Verification items for the finished model (mm, model axes). Face numbers are marked on the shaded views. Coordinates: 2 decimals unless noted, no trailing zeros. Write each loop counter-clockwise with the first axis right and the second up, starting at its lowest first coordinate (ties: lowest second). Pieces come first, ordered by that corner, then holes.
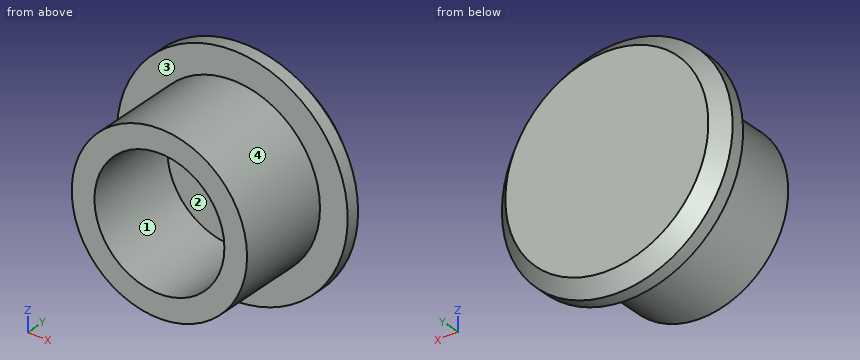
```python
from build123d import *

# Parameters (mm, degrees)
SKETCH1_R           = 6.33
BOSS_EXTRUDE1_DEPTH = 7
SKETCH2_R           = 4.691712698
CUT_EXTRUDE1_DEPTH  = 7
SKETCH3_R           = 8.33
BOSS_EXTRUDE2_DEPTH = 2
CHAMFER1_SIZE       = 1


with BuildPart() as part:
    # Sketch1 → Boss-Extrude1 (new body)
    with BuildSketch(Plane(origin=(0, 0, 0), x_dir=(1, 0, 0), z_dir=(0, 1, 0))):
        Circle(SKETCH1_R)
    extrude(amount=BOSS_EXTRUDE1_DEPTH)

    # Sketch2 → Cut-Extrude1 (cut)
    with BuildSketch(Plane(origin=(0, 7, 0), x_dir=(1, 0, 0), z_dir=(0, 1, 0))):
        Circle(SKETCH2_R)
    extrude(amount=-CUT_EXTRUDE1_DEPTH, mode=Mode.SUBTRACT)

    # Sketch3 → Boss-Extrude2 (add)
    with BuildSketch(Plane(origin=(0, 7, 0), x_dir=(1, 0, 0), z_dir=(0, 1, 0))):
        Circle(SKETCH3_R)
    extrude(amount=BOSS_EXTRUDE2_DEPTH)

    # Chamfer1
    chamfer1_edges = [part.edges().sort_by_distance(p)[0] for p in [
        (-8.33, 9, 0),
    ]]
    chamfer(chamfer1_edges, length=CHAMFER1_SIZE)


solid = part.part
```
1. Sectioned sample at C-C, the plane y = 3.5. Record the boundary of the cut face in (x, z).
2. Sectioned sample at B-B, the plane z = 0. Record the boundary of the cut face in (x, y).
3. Gauge pin test, flat ends, axial feed: P1, Ø4, axis at x = -3, y = 5.5, coming from the -Z side; P2, Ø4, axis at x = -6.5, y = 7, coming from the +Z side; P3, Ø1, axis at y = 3.5, z = -2, coming from the -X side. Record the tip position at first contact, or that the pin passes through.
4. Material ranges on L1, parallel to Z at x = 0, y = 4.75; L2, parallel to Y at x = -0.75, z = -6.5, recorded low to high.
5. Sectioned sample at A-A, the plane x = 0. Record the boundary of the cut face in (y, z), and give its area (3 significant figures).
6. Draft check along Z on the marked faces 1, 2, 3 and 4. Enter one of: pulls with the +Z half, pulls with the -Z half, needs draft (parallel to the pull), parting line crosses it, or undercut.
Outcome:
1. outline: circle Ø12.66 at (0, 0); hole circle Ø9.38 at (0, 0)
2. outline: (-8.33, 7) - (-6.33, 7) - (-6.33, 0) - (-4.69, 0) - (-4.69, 7) - (4.69, 7) - (4.69, 0) - (6.33, 0) - (6.33, 7) - (8.33, 7) - (8.33, 8) - (7.33, 9) - (-7.33, 9) - (-8.33, 8) - close
3. P1: stops at z = -8.16
3. P2: stops at z = 7.01
3. P3: stops at x = -6.15
4. L1: z = -6.33 to -4.69, 4.69 to 6.33
4. L2: y = 7 to 9
5. outline: (0, -6.33) - (7, -6.33) - (7, -8.33) - (8, -8.33) - (9, -7.33) - (9, 7.33) - (8, 8.33) - (7, 8.33) - (7, 6.33) - (0, 6.33) - (0, 4.69) - (7, 4.69) - (7, -4.69) - (0, -4.69) - close
5. area: 55.3 mm2
6. face 1: undercut
6. face 2: undercut
6. face 3: needs draft
6. face 4: parting line crosses it
